The listing builds one solid part. Answer for the finished solid, in the listing's coordinates (mm). A direction names the side the tool comes from. Round coordinates to 2 decimals unless told otherwise and drop trailing zeros. Order: outer loops, then holes, each group sorted by start corner. A loop starts at its lowest first (then second) coordinate and runs counter-clockwise, first axis right, second up. Notation, with made-up numbers: M 58.5,38.25 L 73.5,38.25 A30 ccw 73.5,76.25 Z; hole C 52,-13.5 d8. An arc over 180 degrees is marked long. Write item = value, one per line. Start each with the question number.
(1) Each of these flat-tipped pins is pushed along its axis until it touches: pin 1 (2 mm diameter, centred on x = -53.5, z = -12, fed in from -Y); pin 2 (3 mm diameter, centred on x = 59.5, z = -110, fed in from -Y); pin 3 (4 mm diameter, centred on y = -338.62, z = -30.19, fed in from +X); pin 4 (5 mm diameter, centred on y = -332.99, z = -25.46, fed in from -X). Where does it stop, or does it pass through?
(2) For a pull along Z with two mould halves and no side action, classify faces 4 (the face through (40, -300, -61)), 5 (the face through (-30, -242, 0)), 6 (the face through (-35.07, -312.73, -61.63)) as released by +Z, released by -Z, zero draft, split by the parting line, or undercut.
(3) A cutting plane is placed at B-B, the plane y = -272.5. Determine the outline of the cut face in (x, z).
(4) Which of the six approach directions +Z, -Z, +X, -X, +Y, -Y give full straight-line access (tool end or side, diameter ignored) to faces 1 (the face through (0, -248.803, -61)), 2 (the face through (-57, -211, -10)), 3 (the face through (34.93, -293.85, -12.34))?
(5) Straight lines are drawn through the part: probe 1 along Z at (x, y) = (-60, -211.45); probe 2 along X at (y, z) = (-320.5, -83); probe 3 along Y at (x, z) = (8.5, -7.5). For each, find the intervals that lie inside material, in ascending order. Write a range as from..to.
from build123d import *

# Parameters (mm, degrees)
BOSS_EXTRUDE1_DEPTH = 120
SKETCH2_W           = 80
SKETCH2_H           = 30
BOSS_EXTRUDE2_DEPTH = 120
FILLET1_R           = 20
SKETCH3_W           = 10
SKETCH3_H           = 120
BOSS_EXTRUDE3_DEPTH = 120
FILLET2_R           = 60
SKETCH4_R           = 4.25
SKETCH4_R_2         = 2.25
CUT_EXTRUDE1_DEPTH  = 406.975263542
SKETCH6_W           = 20
SKETCH6_H           = 17
SKETCH6_W_2         = 16
SKETCH6_H_2         = 13
BOSS_EXTRUDE4_DEPTH = 20
SKETCH7_W           = 20
SKETCH7_H           = 17
BOSS_EXTRUDE5_DEPTH = 3
FILLET3_R           = 13
SKETCH8_R           = 6
CUT_EXTRUDE2_DEPTH  = 3
CHAMFER1_SIZE       = 17
SKETCH10_R          = 1.65
CUT_EXTRUDE3_DEPTH  = 218.122958345
SKETCH11_R          = 3
CUT_EXTRUDE4_DEPTH  = 215.149368903
BOSS_EXTRUDE6_DEPTH = 10
CHAMFER3_SIZE       = 17


with BuildPart() as part:
    # Sketch1 → Boss-Extrude1 (new body)
    with BuildSketch(Plane.XY):
        with BuildLine():
            Line((80, -206.5), (-80, -206.5))
            Line((-80, -206.5), (-80, -206.771199773))
            ThreePointArc((-80, -206.771199773), (-65.350122978, -210.451524762), (-51.0095809, -215.196263078))
            ThreePointArc((-51.0095809, -215.196263078), (0, -224.378994833), (51.0095809, -215.196263078))
            ThreePointArc((51.0095809, -215.196263078), (65.350122978, -210.451524762), (80, -206.771199773))
            Line((80, -206.771199773), (80, -206.5))
        make_face()
    extrude(amount=-BOSS_EXTRUDE1_DEPTH)

    # Sketch2 → Boss-Extrude2 (add)
    with BuildSketch(Plane(origin=(0, 0, -120), x_dir=(-1, 0, 0), z_dir=(0, 0, -1))):
        with Locations((0, -233.803354766)):
            Rectangle(SKETCH2_W, SKETCH2_H)
    extrude(amount=-BOSS_EXTRUDE2_DEPTH)

    # Fillet1
    fillet1_edges = [part.edges().sort_by_distance(p)[0] for p in [
        (40, -218.803354766, -60),
        (-40, -218.803354766, -60),
    ]]
    fillet(fillet1_edges, radius=FILLET1_R)

    # Sketch3 → Boss-Extrude3 (add)
    with BuildSketch(Plane.XZ.offset(248.803354766)):
        with Locations((35, -60)):
            Rectangle(SKETCH3_W, SKETCH3_H)
        with Locations((-35, -60)):
            Rectangle(SKETCH3_W, SKETCH3_H)
    extrude(amount=BOSS_EXTRUDE3_DEPTH)

    # Fillet2
    fillet2_edges = [part.edges().sort_by_distance(p)[0] for p in [
        (35, -368.803354766, -120),
        (35, -368.803354766, 0),
        (-35, -368.803354766, 0),
        (-35, -368.803354766, -120),
    ]]
    fillet(fillet2_edges, radius=FILLET2_R - 0.0001)  # a hair under: the kernel refuses the full size

    # Sketch4 → Cut-Extrude1 (cut, through all)
    with BuildSketch(Plane.ZY.offset(40)):
        with Locations(Location((-60, -308.803354766, 0), (0, 0, 270))):
            Circle(SKETCH4_R)
        with Locations(Location((-60, -358.803354766, 0), (0, 0, 270))):
            Circle(SKETCH4_R_2)
        with Locations(Location((-51.317591117, -358.043742416, 0), (0, 0, 270))):
            Circle(SKETCH4_R_2)
        with Locations(Location((-42.898992834, -355.787985805, 0), (0, 0, 270))):
            Circle(SKETCH4_R_2)
        with Locations(Location((-35, -352.104624955, 0), (0, 0, 270))):
            Circle(SKETCH4_R_2)
        with Locations(Location((-27.860619516, -347.105576922, 0), (0, 0, 270))):
            Circle(SKETCH4_R_2)
        with Locations(Location((-21.697777844, -340.94273525, 0), (0, 0, 270))):
            Circle(SKETCH4_R_2)
        with Locations(Location((-16.698729811, -333.803354766, 0), (0, 0, 270))):
            Circle(SKETCH4_R_2)
        with Locations(Location((-13.015368961, -325.904361932, 0), (0, 0, 270))):
            Circle(SKETCH4_R_2)
        with Locations(Location((-10.759612349, -317.485763649, 0), (0, 0, 270))):
            Circle(SKETCH4_R_2)
        with Locations(Location((-10, -308.803354766, 0), (0, 0, 270))):
            Circle(SKETCH4_R_2)
        with Locations(Location((-10.759612349, -300.120945882, 0), (0, 0, 270))):
            Circle(SKETCH4_R_2)
        with Locations(Location((-13.015368961, -291.702347599, 0), (0, 0, 270))):
            Circle(SKETCH4_R_2)
        with Locations(Location((-56.325476132, -350.803354766, 0), (0, 0, 270))):
            Circle(SKETCH4_R_2)
        with Locations(Location((-49.088076944, -349.527206019, 0), (0, 0, 270))):
            Circle(SKETCH4_R_2)
        with Locations(Location((-42.182231017, -347.013683659, 0), (0, 0, 270))):
            Circle(SKETCH4_R_2)
        with Locations(Location((-35.817768983, -343.339159791, 0), (0, 0, 270))):
            Circle(SKETCH4_R_2)
        with Locations(Location((-30.188071803, -338.615282963, 0), (0, 0, 270))):
            Circle(SKETCH4_R_2)
        with Locations(Location((-25.464194975, -332.985585782, 0), (0, 0, 270))):
            Circle(SKETCH4_R_2)
        with Locations(Location((-21.789671107, -326.621123749, 0), (0, 0, 270))):
            Circle(SKETCH4_R_2)
        with Locations(Location((-19.276148747, -319.715277822, 0), (0, 0, 270))):
            Circle(SKETCH4_R_2)
        with Locations(Location((-18, -312.477878634, 0), (0, 0, 270))):
            Circle(SKETCH4_R_2)
        with Locations(Location((-18, -305.128830898, 0), (0, 0, 270))):
            Circle(SKETCH4_R_2)
        with Locations(Location((-19.276148747, -297.89143171, 0), (0, 0, 270))):
            Circle(SKETCH4_R_2)
    extrude(amount=-CUT_EXTRUDE1_DEPTH, mode=Mode.SUBTRACT)

    # Sketch6 → Boss-Extrude4 (add)
    with BuildSketch(Plane(origin=(0, -206.5, 0), x_dir=(1, 0, 0), z_dir=(0, 1, 0))):
        with Locations((0, -8.5)):
            Rectangle(SKETCH6_W, SKETCH6_H)
        with Locations((0, -8.5)):
            Rectangle(SKETCH6_W_2, SKETCH6_H_2, mode=Mode.SUBTRACT)
    extrude(amount=-BOSS_EXTRUDE4_DEPTH)

    # Sketch7 → Boss-Extrude5 (add)
    with BuildSketch(Plane.XZ.offset(226.5)):
        with Locations((0, 8.5)):
            Rectangle(SKETCH7_W, SKETCH7_H)
    extrude(amount=BOSS_EXTRUDE5_DEPTH)

    # Fillet3
    fillet3_edges = [part.edges().sort_by_distance(p)[0] for p in [
        (0, -226.5, 2),
    ]]
    fillet(fillet3_edges, radius=FILLET3_R - 0.0001)  # a hair under: the kernel refuses the full size

    # Sketch8 → Cut-Extrude2 (cut)
    with BuildSketch(Plane.XY.offset(17)):
        with Locations((0, -218)):
            Circle(SKETCH8_R)
    extrude(amount=-CUT_EXTRUDE2_DEPTH, mode=Mode.SUBTRACT)

    # Chamfer1
    chamfer1_edges = [part.edges().sort_by_distance(p)[0] for p in [
        (0, -229.5, 0),
    ]]
    chamfer(chamfer1_edges, length=CHAMFER1_SIZE - 0.0001)  # a hair under: the kernel refuses the full size

    # Sketch10 → Cut-Extrude3 (cut, through all)
    with BuildSketch(Plane(origin=(0, -206.5, 0), x_dir=(1, 0, 0), z_dir=(0, 1, 0))):
        with Locations(Location((-60, 110, 0), (0, 0, 270))):
            Circle(SKETCH10_R)
        with Locations(Location((-60, 10, 0), (0, 0, 270))):
            Circle(SKETCH10_R)
        with Locations(Location((60, 10, 0), (0, 0, 270))):
            Circle(SKETCH10_R)
        with Locations(Location((60, 110, 0), (0, 0, 270))):
            Circle(SKETCH10_R)
    extrude(amount=-CUT_EXTRUDE3_DEPTH, mode=Mode.SUBTRACT)

    # Sketch11 → Cut-Extrude4 (cut, through all)
    with BuildSketch(Plane(origin=(0, -210.5, 0), x_dir=(1, 0, 0), z_dir=(0, 1, 0))):
        with Locations(Location((-60, 110, 0), (0, 0, 270))):
            Circle(SKETCH11_R)
        with Locations(Location((-60, 10, 0), (0, 0, 270))):
            Circle(SKETCH11_R)
        with Locations(Location((60, 110, 0), (0, 0, 270))):
            Circle(SKETCH11_R)
        with Locations(Location((60, 10, 0), (0, 0, 270))):
            Circle(SKETCH11_R)
    extrude(amount=-CUT_EXTRUDE4_DEPTH, mode=Mode.SUBTRACT)

    # Sketch13 → Boss-Extrude6 (add)
    with BuildSketch(Plane.ZY.offset(40)):
        Polygon((-60, -374.803354766), (-63.515300685, -368.700288419), (-60, -366.67551297), (-56.484699315, -368.700288419), align=None)
    extrude(amount=-BOSS_EXTRUDE6_DEPTH)

    # Chamfer3
    chamfer3_edges = [part.edges().sort_by_distance(p)[0] for p in [
        (10, -226.49995, 0),
        (-10, -226.49995, 0),
    ]]
    chamfer(chamfer3_edges, length=CHAMFER3_SIZE - 0.0001)  # a hair under: the kernel refuses the full size


solid = part.part
Reported:
q1.pin_1 = -214.66
q1.pin_2 = -210.5
q1.pin_3 = through
q1.pin_4 = -40
q2.face_4 = zero draft
q2.face_5 = released by +Z
q2.face_6 = undercut
q3.outline = M -40,-120 L -30,-120 L -30,0 L -40,0 Z; M 30,-120 L 40,-120 L 40,0 L 30,0 Z
q4.face_1 = +Z, -Z, -Y
q4.face_2 = -Y
q4.face_3 = +X, -X
q5.probe_1 = -120..-113, -107..-13, -7..0
q5.probe_2 = -40..-30, 30..40
q5.probe_3 = -248.8..-206.5
